from build123d import *

# Parameters (mm, degrees)
EXTRUDE_2_DEPTH = 25
SKETCH_3_W      = 160
SKETCH_3_H      = 25
SKETCH_3_R      = 5
EXTRUDE_3_DEPTH = 25


with BuildPart() as part:
    # 草图1 → 凸台-拉伸2 (new body)
    with BuildSketch(Plane.XY):
        Polygon((0, 0), (0, -40), (-149.841058107, -40), (-322.072943576, 127.48172604), (-244.168859764, 328.224008492), (-225.523676843, 320.988184155), (-289.976254661, 154.907576464), (-130.675150004, 0), align=None)
    extrude(amount=EXTRUDE_2_DEPTH)

    # 草图3 → 凸台-拉伸3 (add)
    with BuildSketch(Plane(origin=(0, 0, 0), x_dir=(-1, 0, 0), z_dir=(0, 0, -1))):
        with Locations((-80, -27.5)):
            Rectangle(SKETCH_3_W, SKETCH_3_H)
        with Locations((-80, -27.5)):
            Circle(SKETCH_3_R, mode=Mode.SUBTRACT)
    extrude(amount=-EXTRUDE_3_DEPTH)


solid = part.part
Could you check a few things on this model? Use its own coordinates, in mm. A direction names the side the tool comes from. Round coordinates to 2 decimals unless told otherwise and drop trailing zeros. Order: outer loops, then holes, each group sorted by start corner. A loop starts at its lowest first (then second) coordinate and runs counter-clockwise, first axis right, second up.
Q1. Please list where these lines run through material, in increasing order: probe 1 along Y at (x, z) = (80, 11.25); probe 2 along Y at (x, z) = (-114.5, 5.5); probe 3 along Y at (x, z) = (119.5, 17.5).
Geometry says:
probe 1: y = -40 to -32.5, -22.5 to -15
probe 2: y = -40 to 0
probe 3: y = -40 to -15
Q2. Imagine slicing it at D-D, the plane x = 7. List the corners of the cut face in (y, z) for me, then the cut area to 3 significant figures.
Geometry says:
outline: (-40, 0) - (-15, 0) - (-15, 25) - (-40, 25) - close
area: 625 mm2
Q3. Thinking about a two-plate mould opening in X: for faces 1 (the face through (-169, 36, 25)), 2 (the face through (0, -7, 12)), 3 (the face through (75.381, -29.415, 12.325)), which applies, released by +X, released by -X, zero draft, split by the parting line, or undercut?
Geometry says:
face 1: zero draft
face 2: released by +X
face 3: undercut
Q4. I'm going to push flat-ended pins straight in: P1, Ø1.5, axis at x = -227, z = 9, coming from the -Y side; P2, Ø4.5, axis at y = -10.5, z = 11.5, coming from the +X side; P3, Ø10, axis at y = 123, z = 11.5, coming from the +X side; P4, Ø16, axis at x = 80, y = -27.5, coming from the +Z side. Where does each tip first touch, or does it pass through?
Geometry says:
P1: stops at y = 34.3
P2: stops at x = 0
P3: stops at x = -252.02
P4: stops at z = 25
Q5. Imagine slicing it at A-A, the plane x = 80. List the corners of the cut face in (y, z) for me, then the cut area to 3 significant figures.
Geometry says:
outline: (-40, 0) - (-32.5, 0) - (-32.5, 25) - (-40, 25) - close; (-22.5, 0) - (-15, 0) - (-15, 25) - (-22.5, 25) - close
area: 375 mm2
Q6. Imagine slicing it at C-C, the plane z = 21. List the corners of the cut face in (x, y) for me.
Geometry says:
outline: (-322.07, 127.48) - (-149.84, -40) - (160, -40) - (160, -15) - (0, -15) - (0, 0) - (-130.68, 0) - (-289.98, 154.91) - (-225.52, 320.99) - (-244.17, 328.22) - close; hole circle Ø10 at (80, -27.5)
Q7. Which directions (+Z, -Z, +X, -X, +Y, -Y) give clear straight access to the entire face, cutting with the end or side of a thin tool? Please do faces 4 (the face through (81, -15, 12)), 5 (the face through (-211.4, 78.5, 12.3)), 6 (the face through (7, -40, 12)).
Geometry says:
face 4: +Z, -Z, +X, +Y
face 5: +Z, -Z, +X
face 6: +Z, -Z, +X, -X, -Y
Q8. Imagine slicing it at B-B, the plane y = -27.5. List the corners of the cut face in (x, z) for me.
Geometry says:
outline: (-162.7, 0) - (75, 0) - (75, 25) - (-162.7, 25) - close; (85, 0) - (160, 0) - (160, 25) - (85, 25) - close
